Autodesk Inventor part; units mm, degrees
ref_plane "YZ Plane" through (0, 0, 0) normal (1, 0, 0) x (0, 1, 0)
ref_plane "XZ Plane" through (0, 0, 0) normal (0, 1, 0) x (-1, 0, 0)
ref_plane "XY Plane" through (0, 0, 0) normal (0, 0, 1) x (1, 0, 0)
sketch "Эскиз1" plane through (0, 0, 0) normal (0, 0, 1) x (1, 0, 0)
  line L0 (8.5, -11.5) -> (-8.5, -11.5)
  line L1 (-11.5, -8.5) -> (-11.5, 8.5)
  line L2 (-8.5, 11.5) -> (8.5, 11.5)
  line L3 (11.5, 8.5) -> (11.5, -8.5)
  line L4 (11.5, -11.5) -> (-11.5, 11.5) construction
  line L5 (-11.5, -11.5) -> (11.5, 11.5) construction
  line L6 (8, -8) -> (-8, -8) construction
  line L7 (-8, -8) -> (-8, 8) construction
  line L8 (-8, 8) -> (8, 8) construction
  line L9 (8, 8) -> (8, -8) construction
  line L10 (8, -8) -> (-8, 8) construction
  line L11 (-8, -8) -> (8, 8) construction
  circle A0 centre (-8, 8) radius 1.75
  circle A1 centre (8, 8) radius 1.75
  circle A2 centre (-8, -8) radius 1.75
  circle A3 centre (8, -8) radius 1.75
  arc A4 (-8.5, 11.5) -> (-11.5, 8.5) centre (-8.5, 8.5) ccw
  arc A5 (11.5, 8.5) -> (8.5, 11.5) centre (8.5, 8.5) ccw
  arc A6 (-11.5, -8.5) -> (-8.5, -11.5) centre (-8.5, -8.5) ccw
  arc A7 (8.5, -11.5) -> (11.5, -8.5) centre (8.5, -8.5) ccw
  line L12 (-9.75, 9.75) -> (9.75, 9.75)
  line L13 (9.75, 9.75) -> (9.75, -9.75)
  line L14 (9.75, -9.75) -> (-9.75, -9.75)
  line L15 (-9.75, -9.75) -> (-9.75, 9.75)
  circle A8 centre (-8, 8) radius 3
  circle A9 centre (8, 8) radius 3
  circle A10 centre (8, -8) radius 3
  circle A11 centre (-8, -8) radius 3
  point P0 (0, 0)
  point P1 (0, 0)
  point P2 (-5.5633, 9.75)
  point P3 (5.5633, 9.75)
  point P4 (9.75, 5.5633)
  point P5 (9.75, -5.5633)
  point P6 (5.5633, -9.75)
  point P7 (-5.5633, -9.75)
  point P8 (-9.75, -5.5633)
  point P9 (-9.75, 5.5633)
  dimension "d0" = 23
  dimension "d2" = 16
  dimension "d4" = 3.5
  dimension "d5" = 3
  dimension "d8" = 6
extrude "Выдавливание1" add sketch "Эскиз1" along normal blind 3.2 contours L0 A6 L1 A4 L2 A5 L3 A7 | A0 L12 A8 L15 | A0 L15 L12 | L12 L15 A8 | A9 L13 L12 | L12 A1 L13 A9 | A11 L14 A2 L15 | L15 L14 A11 | L12 L13 A1 | A2 L14 L15 | A10 L14 L13 | L13 A3 L14 A10 | L13 L14 A3
fillet "Сопряжение1" radius 1.6 8 edges at (5.5633, 9.75, 1.6) (-5.5633, 9.75, 1.6) (-9.75, 5.5633, 1.6) (-9.75, -5.5633, 1.6) (-5.5633, -9.75, 1.6) (5.5633, -9.75, 1.6) (9.75, -5.5633, 1.6) (9.75, 5.5633, 1.6)
chamfer "Фаска1" distance 0.4 angle 45 20 edges at (-9.75, -8, 0) (6.25, -8, 0) (6.25, 8, 0) (-9.75, 8, 0) (0, 9.75, 0) (5.8787, 5.8787, 0) (9.75, 0, 0) (5.8787, -5.8787, 0) (0, -9.75, 0) (-5.8787, -5.8787, 0) (-9.75, 0, 0) (-5.8787, 5.8787, 0) (0, 11.5, 0) (-10.6213, 10.6213, 0) (-11.5, 0, 0) (-10.6213, -10.6213, 0) (0, -11.5, 0) (10.6213, -10.6213, 0) (11.5, 0, 0) (10.6213, 10.6213, 0)
properties part number "Проставка датчика"
Can you work these out from the model? Positions are in its coordinate system, mm. A direction names the side the tool comes from. Round coordinates to 2 decimals unless told otherwise and drop trailing zeros. Loops run counter-clockwise (first coordinate to the right, second up) from the corner with the lowest first, then second, coordinate; pieces in that order, holes last.
Item 1: Suppose I cut it at C-C, the plane z = 2.6. Write out the boundary of the cut face in (x, y).
Item 2: Please list where these lines run through material, in increasing order: L1, parallel to X at y = 8, z = 1.95; L2, parallel to Y at x = 0.75, z = 0.55.
Item 3: Which directions (+Z, -Z, +X, -X, +Y, -Y) give clear straight access to the entire face, cutting with the end or side of a thin tool? Please do faces 4 (the cylindrical face through (-4.565, -9.25, 1.82)), 5 (the cylindrical face through (-10.6, -10.64, 1.78)).
Item 4: Suppose I cut it at A-A, the plane x = -2.5. Write out the boundary of the cut face in (y, z), then the cut area to 3 significant figures.
Item 5: If we mould it in two halves opening along X, with no side actions, what happens to faces 1 (the cylindrical face through (-10.64, 10.6, 1.78)), 2 (the cylindrical face through (10.6, 10.64, 1.78)), 3 (the cylindrical face through (-6.331, -8.526, 1.78))? For each: +X half, -X half, draft (parallel to the pull), parting line (faces both ways), or undercut.
Item 6: Suppose I cut it at D-D, the plane y = -7. State how many separate pieces and enclosed holes the cut face has, then the cut area to 3 significant figures.
Reported:
1. outline: (-11.5, -8.5) arc R3 ccw to (-8.5, -11.5) - (8.5, -11.5) arc R3 ccw to (11.5, -8.5) - (11.5, 8.5) arc R3 ccw to (8.5, 11.5) - (-8.5, 11.5) arc R3 ccw to (-11.5, 8.5) - close; hole circle Ø3.5 at (-8, -8); hole (-9.75, -3.4) arc R1.6 ccw to (-8.1, -5) arc R3 cw to (-5, -8.1) arc R1.6 ccw to (-3.4, -9.75) - (3.4, -9.75) arc R1.6 ccw to (5, -8.1) arc R3 cw to (8.1, -5) arc R1.6 ccw to (9.75, -3.4) - (9.75, 3.4) arc R1.6 ccw to (8.1, 5) arc R3 cw to (5, 8.1) arc R1.6 ccw to (3.4, 9.75) - (-3.4, 9.75) arc R1.6 ccw to (-5, 8.1) arc R3 cw to (-8.1, 5) arc R1.6 ccw to (-9.75, 3.4) - close; hole circle Ø3.5 at (-8, 8); hole circle Ø3.5 at (8, -8); hole circle Ø3.5 at (8, 8)
2. L1: x = -11.5 to -9.75, -6.25 to -5, 5 to 6.25, 9.75 to 11.5
2. L2: y = -11.5 to -9.75, 9.75 to 11.5
3. face 4: +Z, -Z
3. face 5: +Z, -Z, -X, -Y
4. outline: (-11.5, 0.4) - (-11.1, 0) - (-10.15, 0) - (-9.75, 0.4) - (-9.75, 3.2) - (-11.5, 3.2) - close; (9.75, 0.4) - (10.15, 0) - (11.1, 0) - (11.5, 0.4) - (11.5, 3.2) - (9.75, 3.2) - close
4. area: 10.9 mm2
5. face 1: -X half
5. face 2: +X half
5. face 3: undercut
6. separate pieces: 4
6. enclosed holes: 0
6. area: 21.4 mm2
